Build history of the part. All positions in model axes, mm. Face numbers are marked on the shaded views. A direction names the side the tool comes from. Give positions to 0.01 mm unless a question says otherwise; leave off trailing zeros. Loops run counter-clockwise (first coordinate to the right, second up) from the corner with the lowest first, then second, coordinate; pieces in that order, holes last. Notation, with made-up numbers: M 30.25,52 L 76.25,52 A13 cw 76.25,72 Z; hole C 73.25,-36.75 d6. An arc over 180 degrees is marked long. Answer as a JSON object with one key per item and string values. Group by question number.
1. Slice it at A-A (y = 1). List the corners of the cut face in (x, z).
2. Slice it at B-B (z = 0). List the corners of the cut face in (x, y), then the cut area to 3 significant figures.
3. Slice it at D-D (y = 0.7). List the corners of the cut face in (x, z), then the cut area to 3 significant figures.
4. Drop a flat-ended pin along its axis: pin 1 Ø0.6 at (x, z) = (2.5, 2) entering from +Y. Give the stop position or say it passes through.
5. 3-axis set-ups, long thin cutter, end or side, ignore diameter. For the marked faces 1 and 2: which of +Z, -Z, +X, -X, +Y, -Y reach the whole face in a straight line?
6. Drill centre lines: line 1 along X through (y, z) = (0.55, -1.6); line 2 along Y through (x, z) = (1, -1.75); line 3 along X through (y, z) = (1, -1.4). Where is each one in solid material? Low to high. Write a range as [from, to].
7. Slice it at C-C (x = 0). List the corners of the cut face in (y, z), then the cut area to 3 significant figures.
from build123d import *

# Parameters (mm, degrees)
EXTRUDE1_DEPTH = 0.4
EXTRUDE2_DEPTH = 0.8
EXTRUDE3_DEPTH = 1.2
SKETCH4_R      = 1.5
EXTRUDE7_DEPTH = 1.5


with BuildPart() as part:
    # Sketch1 → Extrude1 (new body)
    with BuildSketch(Plane(origin=(0, 0, 0), x_dir=(1, 0, 0), z_dir=(0, 1, 0))):
        Polygon((-3.2, 2.1), (3.2, 2.1), (3.2, 1.6), (2.2, 1.6), (2.2, -1.6), (3.2, -1.6), (3.2, -2.1), (-3.2, -2.1), (-3.2, -1.6), (-2.2, -1.6), (-2.2, 1.6), (-3.2, 1.6), align=None)
    extrude(amount=EXTRUDE1_DEPTH)

    # Sketch2 → Extrude2 (add)
    with BuildSketch(Plane(origin=(0, 0, 0), x_dir=(-1, 0, 0), z_dir=(0, 1, 0))):
        Polygon((1.65, -2.65), (2.65, -1.65), (2.65, 1.65), (1.65, 2.65), (-1.65, 2.65), (-2.65, 1.65), (-2.65, -1.65), (-1.65, -2.65), align=None)
    extrude(amount=EXTRUDE2_DEPTH)

    # Sketch3 → Extrude3 (add)
    with BuildSketch(Plane(origin=(0, 0, 0), x_dir=(-1, 0, 0), z_dir=(0, 1, 0))):
        Polygon((-2.15, 1.442893219), (-2.15, -1.442893219), (-1.442893219, -2.15), (1.442893219, -2.15), (2.15, -1.442893219), (2.15, 1.442893219), (1.442893219, 2.15), (-1.442893219, 2.15), align=None)
    extrude(amount=EXTRUDE3_DEPTH)

    # Sketch4 → Extrude7 (add)
    with BuildSketch(Plane(origin=(0, 0, 0), x_dir=(-1, 0, 0), z_dir=(0, 1, 0))):
        with Locations(Location((0, 0, 0), (0, 0, 90))):  # turned: the seam where the file's is
            Circle(SKETCH4_R)
    extrude(amount=EXTRUDE7_DEPTH)


solid = part.part
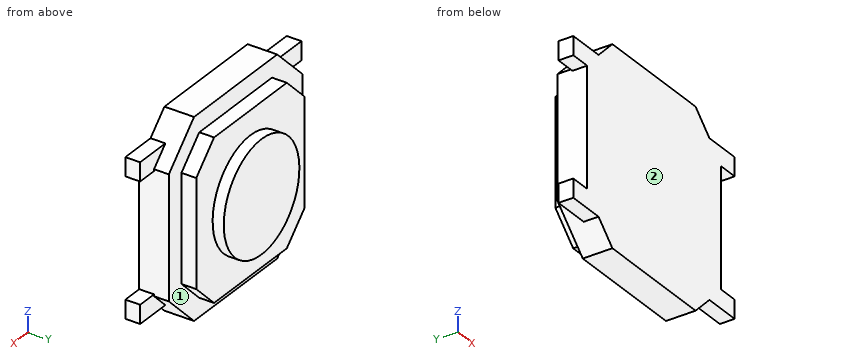
Established:
{
 "1": {"outline": "M -2.15,-1.44 L -1.44,-2.15 L 1.44,-2.15 L 2.15,-1.44 L 2.15,1.44 L 1.44,2.15 L -1.44,2.15 L -2.15,1.44 Z"},
 "2": {"outline": "M -2.65,0 L 2.65,0 L 2.65,0.8 L 2.15,0.8 L 2.15,1.2 L 1.5,1.2 L 1.5,1.5 L -1.5,1.5 L -1.5,1.2 L -2.15,1.2 L -2.15,0.8 L -2.65,0.8 Z", "area": "6.86 mm^2"},
 "3": {"outline": "M -2.65,-1.65 L -1.65,-2.65 L 1.65,-2.65 L 2.65,-1.65 L 2.65,1.65 L 1.65,2.65 L -1.65,2.65 L -2.65,1.65 Z", "area": "26.1 mm^2"},
 "4": {"pin 1": "stops at y = 0.8"},
 "5": {"face 1": "+Y", "face 2": "+Z, -Z, +X, -X, -Y"},
 "6": {"line 1": "x = [-2.65, 2.65]", "line 2": "y = [0, 1.2]", "line 3": "x = [-2.15, 2.15]"},
 "7": {"outline": "M 0,-2.65 L 0.8,-2.65 L 0.8,-2.15 L 1.2,-2.15 L 1.2,-1.5 L 1.5,-1.5 L 1.5,1.5 L 1.2,1.5 L 1.2,2.15 L 0.8,2.15 L 0.8,2.65 L 0,2.65 Z", "area": "6.86 mm^2"}
}
